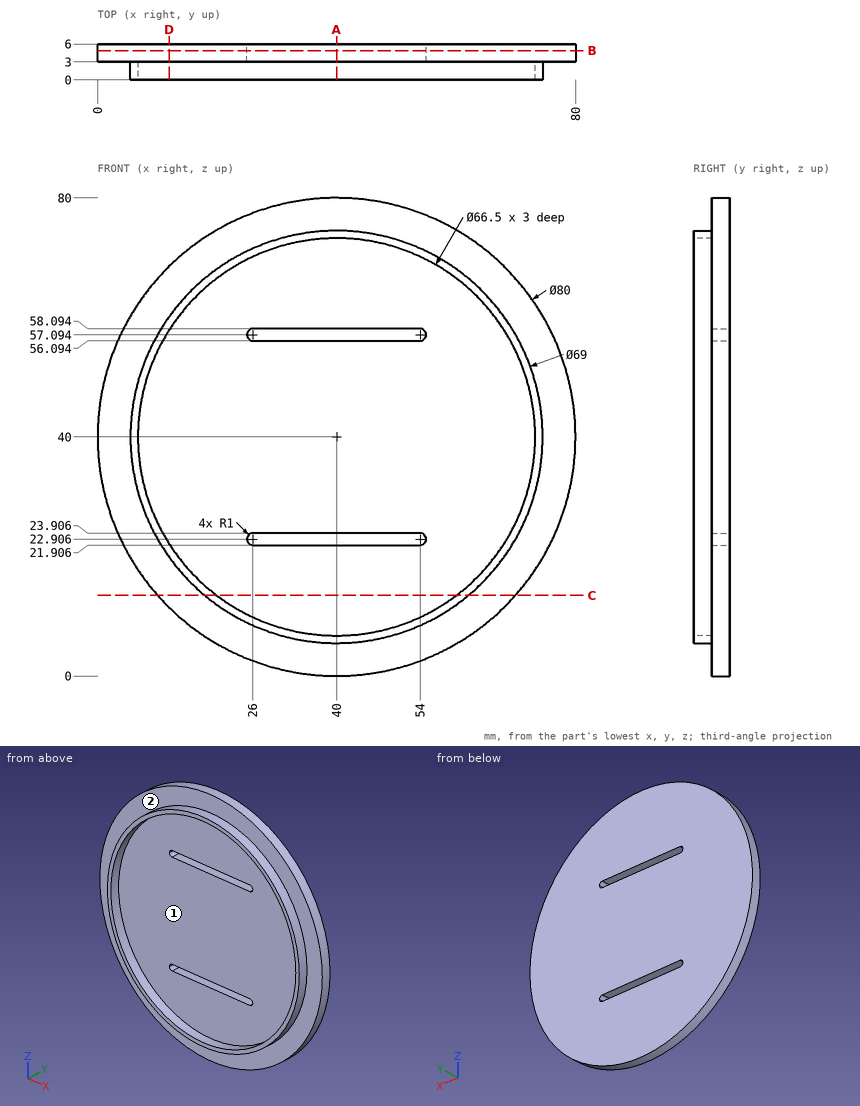
Input: dimensioned drawing with shaded views. Units: mm. Origin: part minimum x, y, z. Coordinates: 2 decimals unless noted, no trailing zeros. Loops run counter-clockwise (first coordinate to the right, second up) from the corner with the lowest first, then second, coordinate; pieces in that order, holes last. Notation, with made-up numbers: M -25.5,44.5 L -5.5,44.5 A21 cw -5.5,79.5 Z; hole C -10.5,21.5 d11. An arc over 180 degrees is marked long. One line per item, written item: value.
(1) Pin query (flat end, axial travel): pin 1 (1.5 mm diameter, centred on x = 42, y = 4, fed in from +Z); pin 2 (2.5 mm diameter, centred on x = 39.5, y = 4.5, fed in from -Z); pin 3 (20 mm diameter, centred on x = 43, z = 55.5, fed in from -Y); pin 4 (4 mm diameter, centred on x = 70, z = 51, fed in from -Y). Return the tip coordinate at first contact, or that it passes through.
Filled in:
pin 1: z = 79.98
pin 2: z = 0
pin 3: y = 3
pin 4: y = 0
(2) Section C-C (z = 13.5). Output: boundary loops of the cut face in (x, y), and give its area (3 significant figures).
Filled in:
outline: M 10.04,3 L 17.91,3 L 17.91,0 L 19.92,0 L 19.92,3 L 60.08,3 L 60.08,0 L 62.09,0 L 62.09,3 L 69.96,3 L 69.96,6 L 10.04,6 Z
area: 192 mm^2
(3) Pull-direction query (Z, two-part tool) for the marked faces 1 and 2; classes: +Z half, -Z half, draft (parallel to the pull), parting line (faces both ways), or undercut.
Filled in:
face 1: undercut
face 2: draft
(4) Line query: line 1 along Z through (x, y) = (40, 1.55); line 2 along Z through (x, y) = (42, 3.5); line 3 along Z through (x, y) = (30.5, 5.1). Output: solid intervals per line, ascending. Write a range as from..to.
Filled in:
line 1: 5.5..6.75, 73.25..74.5
line 2: 0.05..21.91, 23.91..56.09, 58.09..79.95
line 3: 1.14..21.91, 23.91..56.09, 58.09..78.86
(5) Section A-A (x = 40). Output: boundary loops of the cut face in (y, z).
Filled in:
outline: M 0,5.5 L 3,5.5 L 3,0 L 6,0 L 6,21.91 L 3,21.91 L 3,6.75 L 0,6.75 Z; M 0,73.25 L 3,73.25 L 3,58.09 L 6,58.09 L 6,80 L 3,80 L 3,74.5 L 0,74.5 Z; M 3,23.91 L 6,23.91 L 6,56.09 L 3,56.09 Z
(6) Section D-D (x = 12). Output: boundary loops of the cut face in (y, z).
Filled in:
outline: M 0,19.84 L 3,19.84 L 3,11.43 L 6,11.43 L 6,68.57 L 3,68.57 L 3,60.16 L 0,60.16 L 0,57.93 L 3,57.93 L 3,22.07 L 0,22.07 Z
(7) Section B-B (y = 4.9). Output: boundary loops of the cut face in (x, z).
Filled in:
outline: C 40,40 d80; hole M 25,22.91 A1 ccw 26,21.91 L 54,21.91 A1 ccw 55,22.91 A1 ccw 54,23.91 L 26,23.91 A1 ccw Z; hole M 25,57.09 A1 ccw 26,56.09 L 54,56.09 A1 ccw 55,57.09 A1 ccw 54,58.09 L 26,58.09 A1 ccw Z
